Autodesk Inventor part; units mm, degrees
ref_plane "YZ Plane" through (0, 0, 0) normal (1, 0, 0) x (0, 1, 0)
ref_plane "XZ Plane" through (0, 0, 0) normal (0, 1, 0) x (-1, 0, 0)
ref_plane "XY Plane" through (0, 0, 0) normal (0, 0, 1) x (1, 0, 0)
sketch "Sketch1" plane through (0, 0, 0) normal (0, 1, 0) x (-1, 0, 0)
  line L0 (-0.4496, 29.8144) -> (-0.4496, -0.0337)
  line L1 (54.0096, -0.0338) -> (54.0096, 29.8144)
  line L2 (53.5706, 0) -> (53.6221, -0.0838)
  line L3 (53.56, 0) -> (53.5706, 0)
  line L4 (53.56, -0.0837) -> (53.56, 0)
  line L5 (-0.0106, 0) -> (-0.0621, -0.0838)
  line L6 (-0.8993, -0.0972) -> (-0.0106, 0)
  line L7 (53.5706, 0) -> (54.4593, -0.0972)
  line L8 (0, 0) -> (0, -0.0837)
  line L9 (-0.0106, 0) -> (0, 0)
  line L10 (0, 0) -> (53.56, 0)
  line L11 (53.7094, 29.5089) -> (53.5853, 29.9994)
  line L12 (53.56, 29.512) -> (53.7094, 29.5089)
  line L13 (53.56, 30) -> (53.56, 29.512)
  line L14 (-0.1494, 29.5089) -> (-0.0253, 29.9994)
  line L15 (-0.8993, 29.4222) -> (-0.1494, 29.5089)
  line L16 (0, 29.512) -> (0, 30)
  line L17 (-0.1494, 29.5089) -> (0, 29.512)
  line L18 (53.7094, 29.5089) -> (54.4593, 29.4222)
  line L19 (0, 29.512) -> (53.56, 29.512)
  circle A0 centre (26.78, 15) radius 2.6
  circle A1 centre (84.5793, 29) radius 2.6
  circle A2 centre (-31.0193, 29) radius 3.6
  circle A3 centre (91.5793, 29) radius 1.05
  circle A4 centre (84.5793, 36) radius 1.05
  circle A5 centre (84.5793, 22) radius 1.05
  circle A6 centre (77.5793, 29) radius 1.05
  circle A7 centre (-38.0193, 29) radius 1.05
  circle A8 centre (-31.0193, 36) radius 1.05
  circle A9 centre (-31.0193, 22) radius 1.05
  circle A10 centre (-24.0193, 29) radius 1.05
  circle A11 centre (19.78, 15) radius 1.05
  circle A12 centre (26.78, 22) radius 1.05
  circle A13 centre (33.78, 15) radius 1.05
  circle A14 centre (26.78, 8) radius 1.05
  line L20 (53.5853, 29.9994) -> (53.56, 30)
  line L21 (53.6221, -0.0838) -> (53.56, -0.0837)
  line L22 (-0.0621, -0.0838) -> (-0.8993, -0.0972)
  line L23 (-0.0253, 29.9994) -> (-0.8993, 29.4222)
  line L24 (77.602, 36.0383) -> (74.975, 33.6954)
  line L25 (74.975, 33.6954) -> (72.272, 31.7856)
  line L26 (72.272, 31.7856) -> (69.4931, 30.3089)
  line L27 (69.4931, 30.3089) -> (66.6383, 29.2653)
  line L28 (66.6383, 29.2653) -> (63.7075, 28.6549)
  line L29 (63.7075, 28.6549) -> (60.7007, 28.4776)
  line L30 (60.7007, 28.4776) -> (57.618, 28.7333)
  line L31 (57.618, 28.7333) -> (54.4593, 29.4222)
  line L32 (54.4593, -0.0972) -> (53.6221, -0.0838)
  line L33 (-40.5487, 25.8824) -> (-39.4527, 22.5565)
  line L34 (-39.4527, 22.5565) -> (-38.1807, 19.4832)
  line L35 (-38.1807, 19.4832) -> (-36.7234, 16.6331)
  line L36 (-36.7234, 16.6331) -> (-35.0805, 14.0064)
  line L37 (-35.0805, 14.0064) -> (-33.2522, 11.6029)
  line L38 (-33.2522, 11.6029) -> (-31.2384, 9.4228)
  line L39 (-31.2384, 9.4228) -> (-29.0391, 7.4659)
  line L40 (-29.0391, 7.4659) -> (-26.6543, 5.7324)
  line L41 (-26.6543, 5.7324) -> (-24.0841, 4.2221)
  line L42 (-24.0841, 4.2221) -> (-21.3284, 2.9352)
  line L43 (-21.3284, 2.9352) -> (-18.3872, 1.8715)
  line L44 (-18.3872, 1.8715) -> (-15.2606, 1.0312)
  line L45 (-15.2606, 1.0312) -> (-11.9485, 0.4141)
  line L46 (-11.9485, 0.4141) -> (-8.4509, 0.0204)
  line L47 (-8.4509, 0.0204) -> (-4.7678, -0.1501)
  line L48 (-4.7678, -0.1501) -> (-0.8993, -0.0972)
  line L49 (0, 30) -> (-0.0253, 29.9994)
  line L50 (54.4593, -0.0972) -> (58.3278, -0.1501)
  line L51 (58.3278, -0.1501) -> (62.0109, 0.0204)
  line L52 (62.0109, 0.0204) -> (65.5085, 0.4141)
  line L53 (65.5085, 0.4141) -> (68.8206, 1.0312)
  line L54 (68.8206, 1.0312) -> (71.9472, 1.8715)
  line L55 (71.9472, 1.8715) -> (74.8884, 2.9352)
  line L56 (74.8884, 2.9352) -> (77.6441, 4.2221)
  line L57 (77.6441, 4.2221) -> (80.2143, 5.7324)
  line L58 (80.2143, 5.7324) -> (82.5991, 7.4659)
  line L59 (82.5991, 7.4659) -> (84.7984, 9.4228)
  line L60 (84.7984, 9.4228) -> (86.8122, 11.6029)
  line L61 (86.8122, 11.6029) -> (88.6405, 14.0064)
  line L62 (88.6405, 14.0064) -> (90.2834, 16.6331)
  line L63 (90.2834, 16.6331) -> (91.7407, 19.4832)
  line L64 (91.7407, 19.4832) -> (93.0127, 22.5565)
  line L65 (93.0127, 22.5565) -> (94.1087, 25.8824)
  line L66 (54.4593, 29.4222) -> (53.5853, 29.9994)
  line L67 (-0.8993, 29.4222) -> (-4.058, 28.7333)
  line L68 (-4.058, 28.7333) -> (-7.1407, 28.4776)
  line L69 (-7.1407, 28.4776) -> (-10.1475, 28.6549)
  line L70 (-10.1475, 28.6549) -> (-13.0783, 29.2653)
  line L71 (-13.0783, 29.2653) -> (-15.9331, 30.3089)
  line L72 (-15.9331, 30.3089) -> (-18.712, 31.7856)
  line L73 (-18.712, 31.7856) -> (-21.415, 33.6954)
  line L74 (-21.415, 33.6954) -> (-24.042, 36.0383)
  line L75 (0, -0.0837) -> (-0.0621, -0.0838)
  line L76 (53.56, 30) -> (0, 30)
  arc A15 (-24.042, 36.0383) -> (-40.5487, 25.8824) centre (-31.0892, 28.9999) ccw
  arc A16 (94.1087, 25.8824) -> (77.602, 36.0383) centre (84.6492, 28.9999) ccw
  line L77 (53.56, -0.0837) -> (0, -0.0837)
  line L78 (54.4593, 29.4222) -> (54.4593, -0.0972)
  line L79 (-0.8993, -0.0972) -> (-0.8993, 29.4222)
  line L80 (53.56, 0) -> (53.56, 30)
  line L81 (0, 30) -> (0, 0)
  point P0 (0, 0)
extrude "Extrusion1" add sketch "Sketch1" against normal blind 1.5 contours L15 L17 L81 L9 L6 L79 | L79 L48 L47 L46 L45 L44 L43 L42 L41 L40 L39 L38 L37 L36 L35 L34 L33 A15 L74 L73 L72 L71 L70 L69 L68 L67 | L19 L80 L10 L81 | L12 L18 L78 L7 L3 L80 | L31 L30 L29 L28 L27 L26 L25 L24 A16 L65 L64 L63 L62 L61 L60 L59 L58 L57 L56 L55 L54 L53 L52 L51 L50 L78
properties part number "axis_15_bottom_frame"
Model file for the job. Use its own axes, mm. A direction names the side the tool comes from. Give positions to 0.01 mm unless a question says otherwise; leave off trailing zeros. Loops run counter-clockwise (first coordinate to the right, second up) from the corner with the lowest first, then second, coordinate; pieces in that order, holes last.
1) Tool access for faces 1 (the flat face through (-26, 0, 20)), 2 (the flat face through (-76.307, -0.74, 34.883)): list every direction of +Z, -Z, +X, -X, +Y, -Y with a clear straight run to the whole face (end or side of a thin tool).
2) Flat gauge pin, fed straight in: pin 1 Ø0.8 at (x, y) = (-28.5, -0.5) entering from -Z. Where does the tip first touch, or does it go through?
3) Pull direction X, two halves, no side cores. Call faces 3 (the flat face through (-26, -1.5, 20)), 4 (the cylindrical face through (-87.06, -0.74, 29.78)): +X half, -X half, draft (parallel to the pull), parting line (faces both ways), or undercut.
4) Saw through at A-A (y = -1). Count the separate pieces of the cut face and the enclosed holes in it, plus the area to 3 significant figures.
5) Wall check: line 1 (Z direction, x = -26.78, y = -0.95); line 2 (Z direction, x = -33.78, y = -0.6); line 3 (Z direction, x = 1, y = -1.4). Give the ranges that are in metal, low to high.
6) Saw through at B-B (x = -51.5). Write the cut outline in (y, z).
Answer block:
1. face 1: +Z, -Z, +X, -X, +Y
1. face 2: +Z, +Y, -Y
2. pin 1: stops at z = 0
3. face 3: draft
3. face 4: undercut
4. separate pieces: 1
4. enclosed holes: 15
4. area: 3,720 mm2
5. line 1: z = 0 to 6.95, 9.05 to 12.4, 17.6 to 20.95, 23.05 to 29.51
5. line 2: z = 0 to 13.95, 16.05 to 29.51
5. line 3: z = -0.1 to 29.4
6. outline: (-1.5, 0) - (0, 0) - (0, 29.51) - (-1.5, 29.51) - close
